from build123d import *

# Parameters (mm, degrees)
F0_W     = 0.5
F0_H     = 0.5
F1_DEPTH = 3
F2_DEPTH = 18


with BuildPart() as f1:
    # F0 (on Front) → F1 (new body)
    with BuildSketch(Plane.XZ):
        Polygon((-0.8, 0), (0, 0), (0.8, 0.8), (0.8, 3.193335), (0, 3.993335), (-0.8, 3.993335), align=None)
        with Locations((0, 0.75)):
            Rectangle(F0_W, F0_H, mode=Mode.SUBTRACT)
        with Locations((0, 2)):
            Rectangle(F0_W, F0_H, mode=Mode.SUBTRACT)
        with Locations((0, 3.25)):
            Rectangle(F0_W, F0_H, mode=Mode.SUBTRACT)
    extrude(amount=F1_DEPTH)

    # F0 (on Front) → F2 (join)
    with BuildSketch(Plane.XZ):
        with Locations((0, 3.25)):
            Rectangle(F0_W, F0_H)
        with Locations((0, 2)):
            Rectangle(F0_W, F0_H)
        with Locations((0, 0.75)):
            Rectangle(F0_W, F0_H)
    extrude(amount=F2_DEPTH)


solid = f1.part
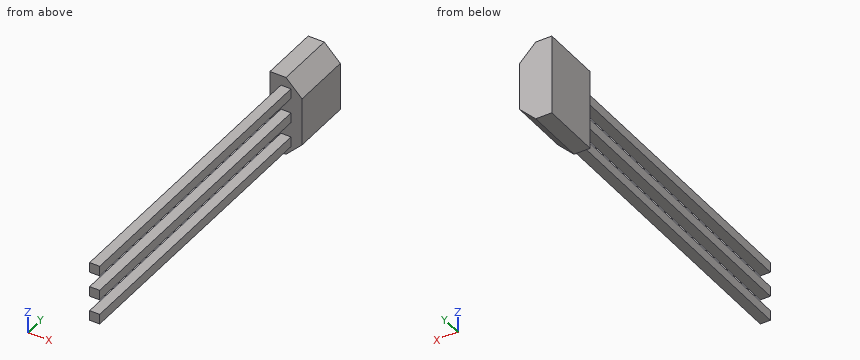
Work out the finished part from the listing and answer in its coordinate system (mm). Round coordinates to 2 decimals unless told otherwise and drop trailing zeros. Write each loop counter-clockwise with the first axis right and the second up, starting at its lowest first coordinate (ties: lowest second). Pieces come first, ordered by that corner, then holes.
1) A cutting plane is placed at A-A (y = -7.25). Give the vertices of the cut face in (x, z).
2) Given pin 1 Ø0.6 at (y, z) = (-10, 1) entering from -X; pin 2 Ø1 at (y, z) = (-16, 1.5) entering from +X, each flat-ended and moving along its own axis, determine where each tip first touches the part or whether it passes through.
3) A cutting plane is placed at C-C (x = -0.4). Give the vertices of the cut face in (y, z), plus the area to 3 significant figures.
4) Straight lines are drawn through the part: line 1 (Z direction, x = 0.1, y = -7); line 2 (Y direction, x = -0.1, z = 2.75); line 3 (X direction, y = -2.75, z = 0.25). For each, find the intervals that lie inside material, in ascending order.
5) A cutting plane is placed at D-D (z = 0.3). Give the vertices of the cut face in (x, y).
6) A cutting plane is placed at B-B (z = 2). Give the vertices of the cut face in (x, y).
Completed:
1. outline: (-0.25, 0.5) - (0.25, 0.5) - (0.25, 1) - (-0.25, 1) - close; (-0.25, 1.75) - (0.25, 1.75) - (0.25, 2.25) - (-0.25, 2.25) - close; (-0.25, 3) - (0.25, 3) - (0.25, 3.5) - (-0.25, 3.5) - close
2. pin 1: stops at x = -0.25
2. pin 2: stops at x = 0.25
3. outline: (-3, 0) - (0, 0) - (0, 3.99) - (-3, 3.99) - close
3. area: 12.0 mm2
4. line 1: z = 0.5 to 1, 1.75 to 2.25, 3 to 3.5
4. line 2: y = -3 to 0
4. line 3: x = -0.8 to 0.25
5. outline: (-0.8, -3) - (0.3, -3) - (0.3, 0) - (-0.8, 0) - close
6. outline: (-0.8, -3) - (-0.25, -3) - (-0.25, -18) - (0.25, -18) - (0.25, -3) - (0.8, -3) - (0.8, 0) - (-0.8, 0) - close
